```python
from build123d import *

# Parameters (mm, degrees)
SKETCH1_R           = 10.5
BOSS_EXTRUDE1_DEPTH = 2
SKETCH2_R           = 4.25
BOSS_EXTRUDE2_DEPTH = 3.5
SKETCH3_R           = 2.75
CUT_EXTRUDE1_DEPTH  = 4.5
SKETCH4_R           = 1.6
CUT_EXTRUDE2_DEPTH  = 3.5
SKETCH5_R           = 1
CUT_EXTRUDE3_DEPTH  = 3.5
CUT_EXTRUDE4_DEPTH  = 4.5
CIRPATTERN1_COUNT   = 25


with BuildPart() as part:
    # Sketch1 → Boss-Extrude1 (new body)
    with BuildSketch(Plane.XY):
        Circle(SKETCH1_R)
    extrude(amount=BOSS_EXTRUDE1_DEPTH)

    # Sketch2 → Boss-Extrude2 (add)
    with BuildSketch(Plane.XY.offset(2)):
        Circle(SKETCH2_R)
    extrude(amount=BOSS_EXTRUDE2_DEPTH)

    # Sketch3 → Cut-Extrude1 (cut)
    with BuildSketch(Plane.XY.offset(5.5)):
        Circle(SKETCH3_R)
    extrude(amount=-CUT_EXTRUDE1_DEPTH, mode=Mode.SUBTRACT)

    # Sketch4 → Cut-Extrude2 (cut)
    with BuildSketch(Plane.XY):
        Circle(SKETCH4_R)
    extrude(amount=CUT_EXTRUDE2_DEPTH, mode=Mode.SUBTRACT)

    # Sketch5 → Cut-Extrude3 (cut)
    with BuildSketch(Plane.XY.offset(2)):
        with Locations((0, 7.4)):
            Circle(SKETCH5_R)
        with Locations((-2.5, 7.4)):
            Circle(SKETCH5_R)
        with Locations((2.5, 7.4)):
            Circle(SKETCH5_R)
        with Locations((2.5, -7.4)):
            Circle(SKETCH5_R)
        with Locations((-2.5, -7.4)):
            Circle(SKETCH5_R)
        with Locations((0, -7.4)):
            Circle(SKETCH5_R)
        with Locations((7.4, 0)):
            Circle(SKETCH5_R)
        with Locations((7.4, 2.5)):
            Circle(SKETCH5_R)
        with Locations((7.4, -2.5)):
            Circle(SKETCH5_R)
        with Locations((-7.4, -2.5)):
            Circle(SKETCH5_R)
        with Locations((-7.4, 2.5)):
            Circle(SKETCH5_R)
        with Locations((-7.4, 0)):
            Circle(SKETCH5_R)
    extrude(amount=-CUT_EXTRUDE3_DEPTH, mode=Mode.SUBTRACT)

    # Sketch6 → Cut-Extrude4 (cut)
    with BuildSketch(Plane.XY.offset(5.5)):
        with BuildLine():
            Line((-2.895429002, 0.78516934), (-2.654143252, 0.719738562))
            ThreePointArc((-2.654143252, 0.719738562), (-2.605253752, 0.880427673), (-2.546645605, 1.037832435))
            Line((-2.546645605, 1.037832435), (-2.895429002, 0.78516934))
        make_face()
        with BuildLine():
            Line((-2.895429002, 0.78516934), (-2.723421701, 0.381410852))
            ThreePointArc((-2.723421701, 0.381410852), (-2.694098665, 0.551663288), (-2.654143252, 0.719738562))
            Line((-2.654143252, 0.719738562), (-2.895429002, 0.78516934))
        make_face()
    cut_extrude4 = extrude(amount=-CUT_EXTRUDE4_DEPTH, mode=Mode.SUBTRACT)

    # CirPattern1: Cut-Extrude4 ×25 about axis
    cirpattern1_axis = Axis((0, 0, 0), (0, 0, 1))
    for i in range(1, CIRPATTERN1_COUNT):
        add(cut_extrude4.rotate(cirpattern1_axis, i * 360 / CIRPATTERN1_COUNT), mode=Mode.SUBTRACT)


solid = part.part
```
CAD build for the part. Positions are in the model's coordinates, mm. A direction names the side the tool comes from. Round coordinates to 2 decimals unless told otherwise and drop trailing zeros. Order: outer loops, then holes, each group sorted by start corner. A loop starts at its lowest first (then second) coordinate and runs counter-clockwise, first axis right, second up. Notation, with made-up numbers: (57.25, 25) - (105.25, 25) arc R12 cw to (105.25, 48) - close; hole circle Ø2 at (-6, 3.5). An arc over 180 degrees is marked (long way). Use CSV: the item, a comma, the result in double quotes. Start each with the question number.
1) Saw through at B-B (x = 7.25). List the corners of the cut face in (y, z), and give its area (3 significant figures).
2) Saw through at A-A (y = -7.4). List the corners of the cut face in (x, z).
3) Tool access for faces 1 (the cylindrical face through (2.285, 3.584, 3.726)), 2 (the cylindrical face through (-6.94, -0.89, 1.01)): list every direction of +Z, -Z, +X, -X, +Y, -Y with a clear straight run to the whole face (end or side of a thin tool).
4) Pin check, flat tips, straight feed: pin 1 Ø3 at (x, y) = (-7.4, 2.5) entering from +Z; pin 2 Ø1 at (x, z) = (0.5, 1) entering from -Y; pin 3 Ø1.8 at (x, y) = (1, -1) entering from +Z; pin 4 Ø1 at (y, z) = (-4, 2) entering from +X. Stop position of each tip, or through.
5) Wall check: L1, parallel to Y at x = 7.4, z = 0.7; L2, parallel to X at y = 0.5, z = 1.2; L3, parallel to Y at x = 7, z = 1.4. Give the ranges that are in metal, low to high. Write a range as [from, to].
6) Two-plate mould, pull along X, no slides. Class faces 3 (the flat face through (2, 0, 0)), 4 (the cylindrical face through (-6.446, 2.8, 1.014)), 5 (the cylindrical face through (10, 3.2, 1)), 6 (the cylindrical face through (-1.27, -0.97, 0.49)): pulls with the +X half, pulls with the -X half, needs draft (parallel to the pull), parting line crosses it, or undercut.
Values follow:
1,outline,"(-7.6, 0) - (-3.49, 0) - (-3.49, 2) - (-7.6, 2) - close; (-1.51, 0) - (-0.99, 0) - (-0.99, 2) - (-1.51, 2) - close; (0.99, 0) - (1.51, 0) - (1.51, 2) - (0.99, 2) - close; (3.49, 0) - (7.6, 0) - (7.6, 2) - (3.49, 2) - close"
1,area,"18.5 mm2"
2,outline,"(-7.45, 0) - (-3.5, 0) - (-3.5, 2) - (-7.45, 2) - close; (-1.5, 0) - (-1, 0) - (-1, 2) - (-1.5, 2) - close; (1, 0) - (1.5, 0) - (1.5, 2) - (1, 2) - close; (3.5, 0) - (7.45, 0) - (7.45, 2) - (3.5, 2) - close"
3,face 1,"+Z"
3,face 2,"+Z, -Z"
4,pin 1,"stops at z = 2"
4,pin 2,"stops at y = -10.5"
4,pin 3,"stops at z = 1"
4,pin 4,"stops at x = 9.9"
5,L1,"y = [-7.45, -3.5], [-1.5, -1], [1, 1.5], [3.5, 7.45]"
5,L2,"x = [-10.49, -8.27], [-6.53, -2.77], [2.82, 6.53], [8.27, 10.49]"
5,L3,"y = [-7.83, -3.42], [-1.58, -0.92], [0.92, 1.58], [3.42, 7.83]"
6,face 3,"needs draft"
6,face 4,"undercut"
6,face 5,"parting line crosses it"
6,face 6,"undercut"
